```python
from build123d import *

# Parameters (mm, degrees)
F0_W     = 152.4
F0_H     = 152.4
F1_DEPTH = 38.1
F2_W     = 38.1
F2_H     = 38.1
F3_DEPTH = 2514.092
F4_W     = 152.4
F4_H     = 152.4
F5_DEPTH = 38.1
F6_R     = 19.05
F7_DEPTH = 0.254
F8_R     = 19.05
F9_DEPTH = 0.254


with BuildPart() as f1:
    # F0 (on Top) → F1 (new body)
    with BuildSketch(Plane.XY):
        Rectangle(F0_W, F0_H)
    extrude(amount=-F1_DEPTH)

    # F2 (on face) → F3 (join)
    with BuildSketch(Plane.XY):
        with Locations((57.15, -57.15)):
            Rectangle(F2_W, F2_H)
        with Locations((57.15, 57.15)):
            Rectangle(F2_W, F2_H)
        with Locations((-57.15, -57.15)):
            Rectangle(F2_W, F2_H)
        with Locations((-57.15, 57.15)):
            Rectangle(F2_W, F2_H)
    extrude(amount=F3_DEPTH)

    # F4 (on face) → F5 (join)
    with BuildSketch(Plane.XY.offset(2514.092)):
        Rectangle(F4_W, F4_H)
    extrude(amount=F5_DEPTH)

    # F6 (on face) → F7 (cut)
    with BuildSketch(Plane(origin=(0, 0, -38.1), x_dir=(1, 0, 0), z_dir=(0, 0, -1))):
        Circle(F6_R)
    extrude(amount=-F7_DEPTH, mode=Mode.SUBTRACT)

    # F8 (on face) → F9 (cut)
    with BuildSketch(Plane.XY.offset(2552.192)):
        Circle(F8_R)
    extrude(amount=-F9_DEPTH, mode=Mode.SUBTRACT)


solid = f1.part
```
The listing builds one solid part. Answer for the finished solid, in the listing's coordinates (mm). A direction names the side the tool comes from. Round coordinates to 2 decimals unless told otherwise and drop trailing zeros. Write each loop counter-clockwise with the first axis right and the second up, starting at its lowest first coordinate (ties: lowest second). Pieces come first, ordered by that corner, then holes. Notation, with made-up numbers: (-29, 89.25) -> (5, 89.25) arc R19 ccw to (5, 118.25) -> close; hole circle Ø8 at (21.25, -2.75). An arc over 180 degrees is marked (long way). Use CSV: the item, a comma, the result in double quotes. Start each with the question number.
(1) The mould has two halves that part along X. Classify faces 3 (the face through (-1, 1, 0)), 4 (the face through (16, 18, 2552.192)), 5 (the face through (-76.2, -52, 1239)): released by +X, released by -X, zero draft, split by the parting line, or undercut.
(2) Consider L1, parallel to Y at x = 0, z = 2552.1; L2, parallel to X at y = 60, z = 1504.5; L3, parallel to Z at x = -63, y = -22. Determine where each line is inside the solid, lowest interval first. Write a range as from..to.
(3) Section A-A on z = 975.5 is taken. Give the vertices of the cut face in (x, y), then the cut area to 3 significant figures.
(4) Which of the six approach directions +Z, -Z, +X, -X, +Y, -Y give full straight-line access (tool end or side, diameter ignored) to faces 1 (the face through (-1, 1, 2514.092)), 2 (the face through (-52, -76.2, 1239))?
A:
1,face 3,"undercut"
1,face 4,"zero draft"
1,face 5,"released by -X"
2,L1,"y = -76.2..-19.05, 19.05..76.2"
2,L2,"x = -76.2..-38.1, 38.1..76.2"
2,L3,"z = -38.1..0, 2514.09..2552.19"
3,outline,"(-76.2, -76.2) -> (-38.1, -76.2) -> (-38.1, -38.1) -> (-76.2, -38.1) -> close; (-76.2, 38.1) -> (-38.1, 38.1) -> (-38.1, 76.2) -> (-76.2, 76.2) -> close; (38.1, -76.2) -> (76.2, -76.2) -> (76.2, -38.1) -> (38.1, -38.1) -> close; (38.1, 38.1) -> (76.2, 38.1) -> (76.2, 76.2) -> (38.1, 76.2) -> close"
3,area,"5,810 mm²"
4,face 1,"none"
4,face 2,"+Z, -Z, +X, -X, -Y"
